```python
from build123d import *

# Parameters (mm, degrees)
SKIZZE2_W                       = 12
SKIZZE2_H                       = 12
SCHNITT_LINEAR_AUSTRAGEN1_DEPTH = 3


with BuildPart() as part:
    # Skizze1 → Rotation1 (revolve)
    with BuildSketch(Plane(origin=(0, 0, 0), x_dir=(0, 0, -1), z_dir=(1, 0, 0)), mode=Mode.PRIVATE) as rotation1_sk:
        with BuildLine():
            Line((4, 0), (4, 1.25))
            Line((4, 1.25), (0, 1.25))
            Line((0, 1.25), (0, 2.0095))
            Line((0, 2.0095), (0.4905, 2.5))
            Line((0.4905, 2.5), (4, 2.5))
            Line((4, 2.5), (4, 3))
            Line((4, 3), (4.346410162, 3.6))
            Line((4.346410162, 3.6), (6.653589838, 3.6))
            Line((6.653589838, 3.6), (7, 3))
            Line((7, 3), (7, 2.9))
            Line((7, 2.9), (8.2, 2.9))
            ThreePointArc((8.2, 2.9), (8.553553391, 2.753553391), (8.7, 2.4))
            Line((8.7, 2.4), (8.7, 1.7415))
            Line((8.7, 1.7415), (19.8, 1.5))
            Line((19.8, 1.5), (19.8, 0))
            Line((19.8, 0), (4, 0))
        make_face()
    revolve(rotation1_sk.sketch.rotate(Axis((0, 0, -19.8), (0, 0, 1)), 270), axis=Axis((0, 0, -19.8), (0, 0, 1)))

    # Skizze2 → Schnitt-Linear austragen1 (cut)
    with BuildSketch(Plane.XY.offset(-4)):
        Rectangle(SKIZZE2_W, SKIZZE2_H)
        Polygon((-3, -1.732050808), (0, -3.464101615), (3, -1.732050808), (3, 1.732050808), (0, 3.464101615), (-3, 1.732050808), align=None, mode=Mode.SUBTRACT)
    extrude(amount=-SCHNITT_LINEAR_AUSTRAGEN1_DEPTH, mode=Mode.SUBTRACT)


solid = part.part
```
Geometry check sheet. Reference: the model listing, model coordinates, mm. A direction names the side the tool comes from. Give positions to 0.01 mm unless a question says otherwise; leave off trailing zeros. Loops run counter-clockwise (first coordinate to the right, second up) from the corner with the lowest first, then second, coordinate; pieces in that order, holes last. Notation, with made-up numbers: M 25.5,32 L 81.5,32 A17 cw 81.5,52 Z; hole C 73,-14 d4. An arc over 180 degrees is marked long. Write item = value, one per line. Start each with the question number.
1. Section check B-B, the plane z = -17. Enter the section's corners in (x, y), plus the area to 3 significant figures.
2. Go/stop test with flat-tipped pins: P1, Ø3, axis at y = -3, z = -11, coming from the -X side; P2, Ø2, axis at y = 2.5, z = -6, coming from the +X side; P3, Ø4, axis at y = -2.5, z = -12.5, coming from the +X side; P4, Ø0.8, axis at x = 0.5, y = 0, coming from the +Z side. Record where each tip stops, or that it passes through.
3. Draft check along Y on faces 1 (the face through (1.5, -2.6, -5.5)), 2 (the face through (2.744, 1.575, -4.095)), 3 (the face through (0, 0, -4)). Enter one of: +Y half, -Y half, draft (parallel to the pull), parting line (faces both ways), or undercut.
4. Tool access check on faces 4 (the face through (-0.54, -2.44, -2.27)), 5 (the face through (-0.35, -1.58, -14.33)), 6 (the face through (0, 0, -19.8)). Record the directions out of +Z, -Z, +X, -X, +Y, -Y that give a thin tool (end or side, any length) a straight path to the whole face; none if there is none.
5. Section check A-A, the plane z = -9.25. Enter the section's corners in (x, y), plus the area to 3 significant figures.
6. Thickness scan on probe 1 along Y at (x, z) = (0, -2.65); probe 2 along Z at (x, y) = (-1.5, -1); probe 3 along Z at (x, y) = (0.25, 1). Record the ranges inside material, lowest first.
Values follow:
q1.outline = C 0,0 d3.12
q1.area = 7.65 mm^2
q2.P1 = -0.78
q2.P2 = 3
q2.P3 = 1.58
q2.P4 = -4
q3.face_1 = -Y half
q3.face_2 = +Y half
q3.face_3 = undercut
q4.face_4 = +Z
q4.face_5 = -Z
q4.face_6 = -Z, +X, -X, +Y, -Y
q5.outline = C 0,0 d3.46
q5.area = 9.40 mm^2
q6.probe_1 = -2.5 to -1.25, 1.25 to 2.5
q6.probe_2 = -8.7 to 0
q6.probe_3 = -19.8 to -4
